Part model, mm, in its own coordinate system. Face numbers are marked on the shaded views. A direction names the side the tool comes from. Coordinates: 2 decimals unless noted, no trailing zeros. Loops run counter-clockwise (first coordinate to the right, second up) from the corner with the lowest first, then second, coordinate; pieces in that order, holes last.
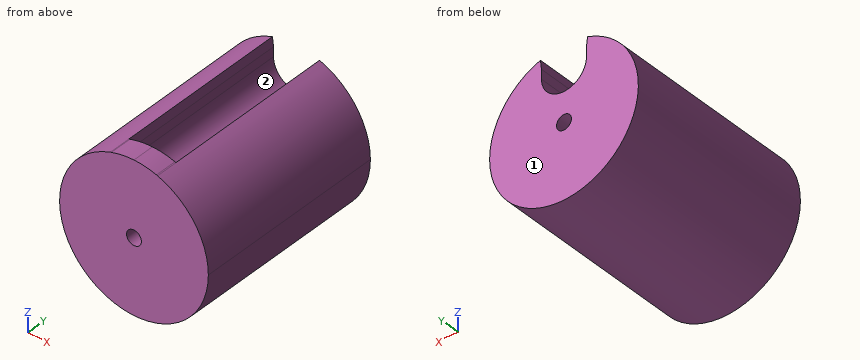
```python
from build123d import *

# Parameters (mm, degrees)
F0_R     = 1.5875
F1_DEPTH = 41.275
F2_DEPTH = 36.576


with BuildPart() as f1:
    # F0 (on Front) → F1 (new body)
    with BuildSketch(Plane.XZ):
        with BuildLine():
            ThreePointArc((-5.031641, 15.056501), (-9.277347, -12.882021), (15.875, 0))
            ThreePointArc((15.875, 0), (12.882021, 9.277347), (5.031641, 15.056501))
            Line((5.031641, 15.056501), (4.8006, 13.103075))
            Line((4.8006, 13.103075), (4.8006, 11.0744))
            ThreePointArc((4.8006, 11.0744), (0, 6.2738), (-4.8006, 11.0744))
            Line((-4.8006, 11.0744), (-4.8006, 13.103075))
            Line((-4.8006, 13.103075), (-5.031641, 15.056501))
        make_face()
        Circle(F0_R, mode=Mode.SUBTRACT)
        with BuildLine():
            Line((4.8006, 13.103075), (4.8006, 15.13175))
            ThreePointArc((4.8006, 15.13175), (2.428898, 15.688087), (0, 15.875))
            ThreePointArc((0, 15.875), (3.394537, 14.468937), (4.8006, 11.0744))
            Line((4.8006, 11.0744), (4.8006, 13.103075))
        make_face()
        with BuildLine():
            ThreePointArc((-4.8006, 15.13175), (-4.916265, 15.094567), (-5.031641, 15.056501))
            Line((-5.031641, 15.056501), (-4.8006, 13.103075))
            Line((-4.8006, 13.103075), (-4.8006, 15.13175))
        make_face()
        with BuildLine():
            ThreePointArc((4.8006, 11.0744), (3.394537, 14.468937), (0, 15.875))
            ThreePointArc((0, 15.875), (-3.394537, 14.468937), (-4.8006, 11.0744))
            ThreePointArc((-4.8006, 11.0744), (0, 6.2738), (4.8006, 11.0744))
        make_face()
        with BuildLine():
            Line((4.8006, 13.103075), (5.031641, 15.056501))
            ThreePointArc((5.031641, 15.056501), (4.916265, 15.094567), (4.8006, 15.13175))
            Line((4.8006, 15.13175), (4.8006, 13.103075))
        make_face()
        with BuildLine():
            ThreePointArc((0, 15.875), (-2.428898, 15.688087), (-4.8006, 15.13175))
            Line((-4.8006, 15.13175), (-4.8006, 13.103075))
            Line((-4.8006, 13.103075), (-4.8006, 11.0744))
            ThreePointArc((-4.8006, 11.0744), (-3.394537, 14.468937), (0, 15.875))
        make_face()
    extrude(amount=F1_DEPTH)

    # F0 (on Front) → F2 (cut)
    with BuildSketch(Plane.XZ):
        with BuildLine():
            ThreePointArc((4.8006, 11.0744), (3.394537, 14.468937), (0, 15.875))
            ThreePointArc((0, 15.875), (-3.394537, 14.468937), (-4.8006, 11.0744))
            ThreePointArc((-4.8006, 11.0744), (0, 6.2738), (4.8006, 11.0744))
        make_face()
        with BuildLine():
            Line((4.8006, 13.103075), (4.8006, 15.13175))
            ThreePointArc((4.8006, 15.13175), (2.428898, 15.688087), (0, 15.875))
            ThreePointArc((0, 15.875), (3.394537, 14.468937), (4.8006, 11.0744))
            Line((4.8006, 11.0744), (4.8006, 13.103075))
        make_face()
        with BuildLine():
            ThreePointArc((0, 15.875), (-2.428898, 15.688087), (-4.8006, 15.13175))
            Line((-4.8006, 15.13175), (-4.8006, 13.103075))
            Line((-4.8006, 13.103075), (-4.8006, 11.0744))
            ThreePointArc((-4.8006, 11.0744), (-3.394537, 14.468937), (0, 15.875))
        make_face()
        with BuildLine():
            ThreePointArc((-4.8006, 15.13175), (-4.916265, 15.094567), (-5.031641, 15.056501))
            Line((-5.031641, 15.056501), (-4.8006, 13.103075))
            Line((-4.8006, 13.103075), (-4.8006, 15.13175))
        make_face()
        with BuildLine():
            Line((4.8006, 13.103075), (5.031641, 15.056501))
            ThreePointArc((5.031641, 15.056501), (4.916265, 15.094567), (4.8006, 15.13175))
            Line((4.8006, 15.13175), (4.8006, 13.103075))
        make_face()
    extrude(amount=F2_DEPTH, mode=Mode.SUBTRACT)


solid = f1.part
```
Q1. Saw through at D-D (z = -4.5). List the corners of the cut face in (x, y) (3 decimals).
Q2. Probe line 1 (Z direction, x = 0, y = -24.5) (1 decimal); line 2 (X direction, y = -5, z = 8); line 3 (X direction, y = -32, z = 14). List the from-to ranges inside material, lowest first.
Q3. Saw through at C-C (z = -9). List the corners of the cut face in (x, y) (3 decimals), plus the area to 3 significant figures.
Q4. Tool access for the marked faces 1 and 2: list every direction of +Z, -Z, +X, -X, +Y, -Y with a clear straight run to the whole face (end or side of a thin tool).
Q5. Drop flat-ended pins along their axis: P1, Ø5, axis at y = -13, z = -3, coming from the -X side; P2, Ø1.5, axis at x = -6, y = -17, coming from the +Z side; P3, Ø10, axis at y = -21.5, z = -9.5, coming from the -X side; P4, Ø5, axis at x = 0, z = 0, coming from the +Y side. Give the stop position or say it passes through.
Q6. Saw through at B-B (x = -2.5). List the corners of the cut face in (y, z) (3 decimals), plus the area to 3 significant figures.
Checked values:
1. outline: (-15.224, -41.275) - (15.224, -41.275) - (15.224, 0) - (-15.224, 0) - close
2. line 1: z = -15.9 to -1.6, 1.6 to 6.3
2. line 2: x = -13.71 to -3.69, 3.69 to 13.71
2. line 3: x = -7.48 to -4.91, 4.91 to 7.48
3. outline: (-13.077, -41.275) - (13.077, -41.275) - (13.077, 0) - (-13.077, 0) - close
3. area: 1,080 mm2
4. face 1: +Z, -Z, +X, -X, +Y
4. face 2: +Z, +Y
5. P1: stops at x = -15.87
5. P2: stops at z = 14.98
5. P3: stops at x = -15.22
5. P4: stops at y = 0
6. outline: (-41.275, -15.677) - (0, -15.677) - (0, 6.976) - (-36.576, 6.976) - (-36.576, 15.677) - (-41.275, 15.677) - close
6. area: 976 mm2
